Can you work these out from the drawing? Everything is in mm from the part's minimum corner. Round coordinates to 2 decimals unless told otherwise and drop trailing zeros. Order: outer loops, then holes, each group sorted by start corner. A loop starts at its lowest first (then second) coordinate and runs counter-clockwise, first axis right, second up. Notation, with made-up numbers: M 72,23 L 89,23 A32 ccw 89,59 Z; hole C 46.25,9 d6. An arc over 180 degrees is marked long. Write each question's results on one line, items separated by ' | '. Start each with the question number.
1. Please list where these lines run through material, in increasing order: L1, parallel to X at y = 2.5, z = 121; L2, parallel to Z at x = 27.5, y = 4.2; L3, parallel to X at y = 1.5, z = 51.5.
2. I'm going to push a flat-ended pin straight in: pin 1 (3 mm diameter, centred on x = 21, y = 3.5, fed in from +Z). Where does the tip first touch, or does it pass through?
3. Suppose I cut it at B-B on y = 4.25. Give the number of separate pieces and of enclosed holes in the cut face, and give its area (3 significant figures).
4. Suppose I cut it at A-A on x = 16. Write out the boundary of the cut face in (y, z), and give its area (3 significant figures).
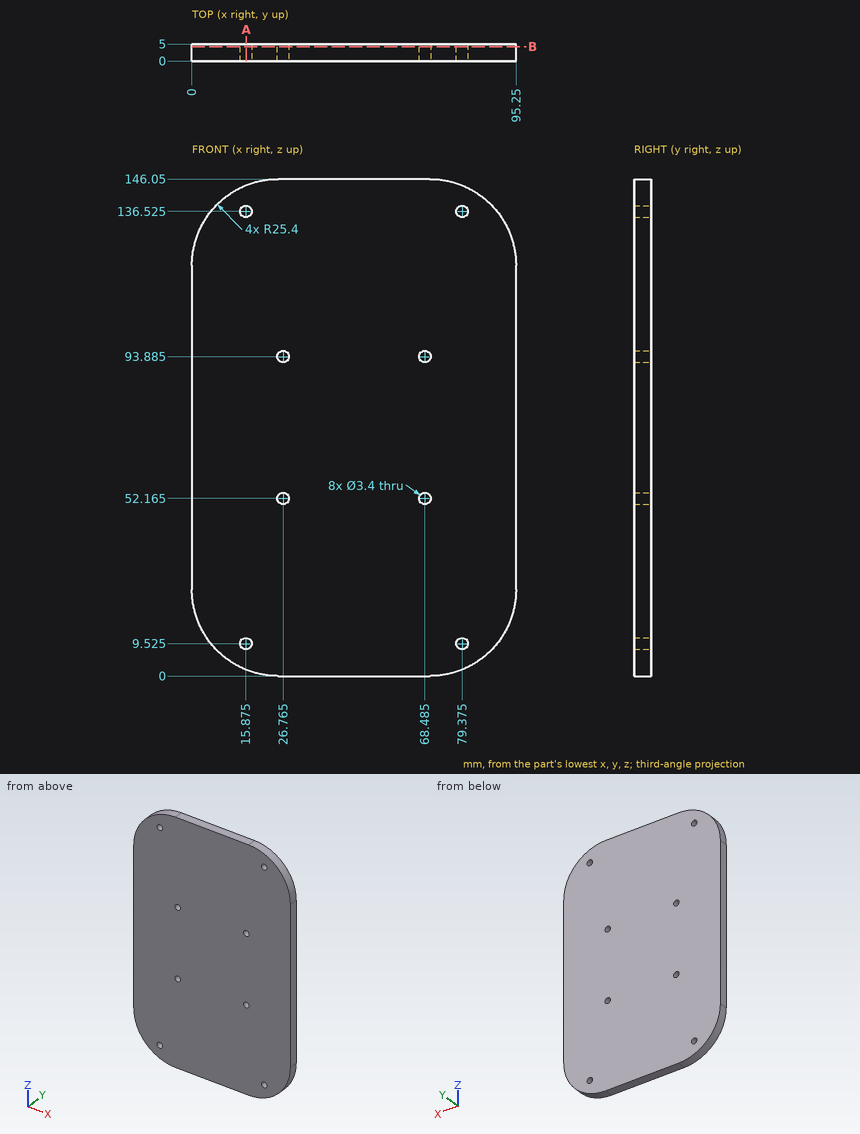
Filled sheet:
1) L1: x = 0 to 95.25 | L2: z = 0 to 50.63, 53.7 to 92.35, 95.42 to 146.05 | L3: x = 0 to 25.2, 28.33 to 66.92, 70.05 to 95.25
2) pin 1: stops at z = 145.88
3) separate pieces: 1 | enclosed holes: 8 | area: 13,300 mm^2
4) outline: M 0,1.8 L 5,1.8 L 5,7.83 L 0,7.83 Z; M 0,11.22 L 5,11.22 L 5,134.83 L 0,134.83 Z; M 0,138.22 L 5,138.22 L 5,144.25 L 0,144.25 Z | area: 678 mm^2
